Check sheet for the modelled part. Datum: model origin and axes. Units: mm. A direction names the side the tool comes from. Give positions to 0.01 mm unless a question says otherwise; leave off trailing zeros. Order: outer loops, then holes, each group sorted by start corner. A loop starts at its lowest first (then second) coordinate and runs counter-clockwise, first axis right, second up. Notation, with made-up numbers: (-38.5, 89) -> (19.5, 89) arc R21 cw to (19.5, 99) -> close; hole circle Ø7 at (62.25, 78). An arc over 180 degrees is marked (long way). One line per question, with ' | ' between items. Start each with the question number.
from build123d import *

# Parameters (mm, degrees)
CROQUIS1_W                 = 6
CROQUIS1_H                 = 35
SALIENTE_EXTRUIR1_DEPTH    = 12.5
CROQUIS2_W                 = 6
CROQUIS2_H                 = 22.5
CORTAR_EXTRUIR1_DEPTH      = 11
CROQUIS3_R                 = 1.5
CORTAR_EXTRUIR2_DEPTH      = 1
CORTAR_EXTRUIR2_DEPTH_BACK = 13.5
CROQUIS4_W                 = 3.5
CROQUIS4_H                 = 4.9
CORTAR_EXTRUIR3_DEPTH      = 1
CORTAR_EXTRUIR3_DEPTH_BACK = 11
CROQUIS5_W                 = 6
CROQUIS5_H                 = 2.5
SALIENTE_EXTRUIR2_DEPTH    = 2.5
CROQUIS6_R                 = 0.6
CORTAR_EXTRUIR4_DEPTH      = 3.7
CORTAR_EXTRUIR4_DEPTH_BACK = 10.8


with BuildPart() as part:
    # Croquis1 → Saliente-Extruir1 (new body)
    with BuildSketch(Plane.XY):
        Rectangle(CROQUIS1_W, CROQUIS1_H)
    extrude(amount=SALIENTE_EXTRUIR1_DEPTH)

    # Croquis2 → Cortar-Extruir1 (cut)
    with BuildSketch(Plane.XY.offset(12.5)):
        Rectangle(CROQUIS2_W, CROQUIS2_H)
    extrude(amount=-CORTAR_EXTRUIR1_DEPTH, mode=Mode.SUBTRACT)

    # Croquis3 → Cortar-Extruir2 (cut, two sides)
    with BuildSketch(Plane(origin=(0, 0, 0), x_dir=(-1, 0, 0), z_dir=(0, 0, -1))) as cortar_extruir2_sk:
        with Locations((0, 5.8)):
            Circle(CROQUIS3_R)
    extrude(amount=CORTAR_EXTRUIR2_DEPTH, mode=Mode.SUBTRACT)
    extrude(cortar_extruir2_sk.sketch, amount=-CORTAR_EXTRUIR2_DEPTH_BACK, mode=Mode.SUBTRACT)

    # Croquis4 → Cortar-Extruir3 (cut, two sides)
    with BuildSketch(Plane.XY.offset(12.5)) as cortar_extruir3_sk:
        with Locations((-1.25, 13.7)):
            Rectangle(CROQUIS4_W, CROQUIS4_H)
        with Locations((-1.25, -13.7)):
            Rectangle(CROQUIS4_W, CROQUIS4_H)
    extrude(amount=CORTAR_EXTRUIR3_DEPTH, mode=Mode.SUBTRACT)
    extrude(cortar_extruir3_sk.sketch, amount=-CORTAR_EXTRUIR3_DEPTH_BACK, mode=Mode.SUBTRACT)

    # Croquis5 → Saliente-Extruir2 (add)
    with BuildSketch(Plane.XZ.offset(-17.5)):
        with Locations((0, 8.55)):
            Rectangle(CROQUIS5_W, CROQUIS5_H)
    extrude(amount=-SALIENTE_EXTRUIR2_DEPTH)

    # Croquis6 → Cortar-Extruir4 (cut, two sides)
    with BuildSketch(Plane.XY.offset(9.8)) as cortar_extruir4_sk:
        with Locations((0, 18.75)):
            Circle(CROQUIS6_R)
    extrude(amount=CORTAR_EXTRUIR4_DEPTH, mode=Mode.SUBTRACT)
    extrude(cortar_extruir4_sk.sketch, amount=-CORTAR_EXTRUIR4_DEPTH_BACK, mode=Mode.SUBTRACT)


solid = part.part
1. Cross-section at B-B on z = 8. Record the boundary of the cut face in (x, y), and give its area (3 significant figures).
2. Go/stop test with flat-tipped pins: pin 1 (3 mm diameter, centred on x = 0.5, y = 18.5, fed in from +Z); pin 2 (0.8 mm diameter, centred on x = 1, y = 19, fed in from -Z); pin 3 (3 mm diameter, centred on x = -1, z = 5.5, fed in from +Y); pin 4 (3 mm diameter, centred on x = 0, y = 1.5, fed in from +Z). Record where each tip stops, or that it passes through.
3. Cross-section at A-A on z = 11.25. Record the boundary of the cut face in (x, y).
4. Cross-section at D-D on x = 0. Record the boundary of the cut face in (y, z), and give its area (4 significant figures).
5. Scan lines: probe 1 along Y at (x, z) = (-0.3, 7); probe 2 along Y at (x, z) = (0, 0.5); probe 3 along Z at (x, y) = (0.35, -14). Record each from-to range of solid material in increasing order.
6. Mould release check, pull along Y, two halves, no side actions. Record for faces 1 (the face through (1, 19, 9.8)), 2 (the face through (-0.078, 19.345, 8.568)), 3 (the face through (0, -17.5, 6)), 4 (the face through (0, 0, 1.5)): +Y half, -Y half, draft (parallel to the pull), parting line (faces both ways), or undercut.
7. Tool access check on faces 5 (the face through (-1, -16.15, 7)), 6 (the face through (1, 19, 7.3)), 7 (the face through (2, -11.25, 7)). Record the directions out of +Z, -Z, +X, -X, +Y, -Y that give a thin tool (end or side, any length) a straight path to the whole face; none if there is none.
8. Cross-section at C-C on y = 5.8. Record the boundary of the cut face in (x, z), and give its area (3 significant figures).
Response values:
1) outline: (-3, -17.5) -> (3, -17.5) -> (3, -11.25) -> (0.5, -11.25) -> (0.5, -16.15) -> (-3, -16.15) -> close; (-3, 16.15) -> (0.5, 16.15) -> (0.5, 11.25) -> (3, 11.25) -> (3, 20) -> (-3, 20) -> close; hole circle Ø1.2 at (0, 18.75) | area: 54.6 mm²
2) pin 1: stops at z = 12.5 | pin 2: stops at z = 7.3 | pin 3: stops at y = 17.5 | pin 4: stops at z = 1.5
3) outline: (-3, -17.5) -> (3, -17.5) -> (3, -11.25) -> (0.5, -11.25) -> (0.5, -16.15) -> (-3, -16.15) -> close; (-3, 16.15) -> (0.5, 16.15) -> (0.5, 11.25) -> (3, 11.25) -> (3, 17.5) -> (-3, 17.5) -> close
4) outline: (-17.5, 0) -> (4.3, 0) -> (4.3, 1.5) -> (-16.15, 1.5) -> (-16.15, 12.5) -> (-17.5, 12.5) -> close; (7.3, 0) -> (17.5, 0) -> (17.5, 7.3) -> (18.15, 7.3) -> (18.15, 9.8) -> (17.5, 9.8) -> (17.5, 12.5) -> (16.15, 12.5) -> (16.15, 1.5) -> (7.3, 1.5) -> close; (19.35, 7.3) -> (20, 7.3) -> (20, 9.8) -> (19.35, 9.8) -> close | area: 80.95 mm²
5) probe 1: y = -17.5 to -16.15, 16.15 to 17.5 | probe 2: y = -17.5 to 4.3, 7.3 to 17.5 | probe 3: z = 0 to 1.5
6) face 1: draft | face 2: undercut | face 3: -Y half | face 4: undercut
7) face 5: +Z, -X | face 6: -Z, +X, -X, +Y | face 7: +Z, +X, -X
8) outline: (-3, 0) -> (-1.5, 0) -> (-1.5, 1.5) -> (-3, 1.5) -> close; (1.5, 0) -> (3, 0) -> (3, 1.5) -> (1.5, 1.5) -> close | area: 4.50 mm²
